Here's how the part is built. I have some questions about the finished solid (model axes, mm). A direction names the side the tool comes from. Round coordinates to 2 decimals unless told otherwise and drop trailing zeros. Loops run counter-clockwise (first coordinate to the right, second up) from the corner with the lowest first, then second, coordinate; pieces in that order, holes last. Notation, with made-up numbers: M 62.25,27.5 L 85.25,27.5 A17 cw 85.25,45.5 Z; hole C 65,21.25 d1. An arc over 180 degrees is marked long. Answer as a JSON object with one key per item and string values.
Autodesk Inventor part; units mm, degrees
ref_plane "YZ Plane" through (0, 0, 0) normal (1, 0, 0) x (0, 1, 0)
ref_plane "XZ Plane" through (0, 0, 0) normal (0, 1, 0) x (-1, 0, 0)
ref_plane "XY Plane" through (0, 0, 0) normal (0, 0, 1) x (1, 0, 0)
sketch "Sketch1" plane through (0, 0, 0) normal (0, 1, 0) x (-1, 0, 0)
  line L0 (-10, -20) -> (10, -20)
  line L1 (10, -20) -> (10, 20)
  line L2 (10, 20) -> (-10, 20)
  line L3 (-10, 20) -> (-10, -20)
  line L4 (-10, -20) -> (10, 20) construction
  line L5 (10, -20) -> (-10, 20) construction
  point P0 (0, 0)
  dimension "d0" = 20
  dimension "d1" = 40
extrude "Extrusion1" add sketch "Sketch1" along normal blind 60
sketch "Sketch2" plane through (0, 0, 0) normal (0, -1, 0) x (1, 0, 0)
  line L0 (10, -20) -> (-10, -20)
  line L1 (10, 20) -> (10, -20)
  line L2 (-10, 20) -> (10, 20)
  line L3 (-10, -20) -> (-10, 20)
  line L4 (10, 20) -> (10, -20)
  line L5 (10, 18.3) -> (-5.8, 18.3)
  line L6 (-5.8, 18.3) -> (-5.8, 16.1)
  line L7 (-5.8, 16.1) -> (10, 16.1)
  line L8 (10, 16.1) -> (10, 18.3)
  point P0 (0, 0)
  dimension "d4" = 1.7
  dimension "d5" = 4.2
  dimension "d6" = 2.2
extrude "Extrusion2" cut sketch "Sketch2" against normal through all contours L7 L6 L5 L1
mirror "Mirror1" about plane through (0, 0, 0) normal (0, 0, 1) of "Extrusion2"
sketch "Sketch3" plane through (0, 0, 0) normal (0, -1, 0) x (1, 0, 0)
  line L0 (-5.8, -16.1) -> (10, -16.1)
  line L1 (10, 16.1) -> (10, -16.1)
  line L2 (10, 16.1) -> (-5.8, 16.1)
  line L3 (-5.8, 16.1) -> (-5.8, 18.3)
  line L4 (-5.8, 18.3) -> (10, 18.3)
  line L5 (10, 20) -> (10, 18.3)
  line L6 (-10, 20) -> (10, 20)
  line L7 (-10, -20) -> (-10, 20)
  line L8 (10, -20) -> (-10, -20)
  line L9 (10, -18.3) -> (10, -20)
  line L10 (10, -18.3) -> (-5.8, -18.3)
  line L11 (-5.8, -18.3) -> (-5.8, -16.1)
  line L12 (10, 14.8) -> (-5.8, 14.8)
  line L13 (-5.8, 14.8) -> (-5.8, 12.28)
  line L14 (-5.8, 12.28) -> (10, 12.28)
  line L15 (10, 12.28) -> (10, 14.8)
  point P0 (0, 0)
  dimension "d9" = 1.3
  dimension "d10" = 2.52
extrude "Extrusion3" cut sketch "Sketch3" against normal through all contours L14 L13 L12 L1
pattern_linear "Rectangular Pattern1" count 8 spacing 3.82 along (0, 0, -1) of "Extrusion3"
sketch "Sketch4" plane through (-10, 0, 20) normal (0, 0, 1) x (1, 0, 0)
  line L0 (-20.7139, 77.7692) -> (45.2661, 77.7692)
  line L1 (45.2661, 77.7692) -> (45.2661, -19.6204)
  line L2 (45.2661, -19.6204) -> (-20.7139, -19.6204)
  line L3 (-20.7139, -19.6204) -> (-20.7139, 77.7692)
  point P0 (10, 0)
extrude "Extrusion4" cut sketch "Sketch4" against normal up to surface (15.36 mm away)
sketch "Sketch5" plane through (10, 0, 4.64) normal (1, 0, 0) x (0, 0, -1)
  line L0 (-2.9581, -8.043) -> (28.5295, -8.043)
  line L1 (28.5295, -8.043) -> (28.5295, 70.3336)
  line L2 (28.5295, 70.3336) -> (-2.9581, 70.3336)
  line L3 (-2.9581, 70.3336) -> (-2.9581, -8.043)
  point P0 (4.64, 0)
extrude "Extrusion5" cut sketch "Sketch5" against normal blind 4
properties part number "Jetson_Heatsink"
Item 1: We'd pull the mould along Z, two halves only. Please class faces 1 (the face through (-3.7, 60, -7.5)), 2 (the face through (0, 30, -0.48)), 3 (the face through (-2, 30, 4.64)), 4 (the face through (-2, 30, -20)): +Z half, -Z half, draft (parallel to the pull), parting line (faces both ways), or undercut.
Solution:
{"face 1": "draft", "face 2": "undercut", "face 3": "+Z half", "face 4": "-Z half"}
Item 2: I want a section at A-A on x = -2.25. List the corners of the cut face in (y, z) for me, plus the area to 3 significant figures.
Solution:
{"outline": "M 0,-20 L 60,-20 L 60,-18.3 L 0,-18.3 Z; M 0,-16.1 L 60,-16.1 L 60,-14.46 L 0,-14.46 Z; M 0,-11.94 L 60,-11.94 L 60,-10.64 L 0,-10.64 Z; M 0,-8.12 L 60,-8.12 L 60,-6.82 L 0,-6.82 Z; M 0,-4.3 L 60,-4.3 L 60,-3 L 0,-3 Z; M 0,-0.48 L 60,-0.48 L 60,0.82 L 0,0.82 Z; M 0,3.34 L 60,3.34 L 60,4.64 L 0,4.64 Z", "area": "590 mm2"}
Item 3: If I drill on L1, parallel to X at y = 52.5, z = -12.5, over which ranges is the centre line in solid material (lowest first)? Write a range as from..to.
Solution:
{"L1": "x = -10..-5.8"}
Item 4: For faces 5 (the face through (6, 30, -19)), 6 (the face through (-5.8, 30, -13)), which set-ups out of +Z, -Z, +X, -X, +Y, -Y let a thin tool reach every point of the face, with its end or its side?
Solution:
{"face 5": "+Z, -Z, +X, +Y, -Y", "face 6": "+X, +Y, -Y"}
Item 5: I want a section at C-C on z = 2.25. List the corners of the cut face in (x, y) for me, plus the area to 3 significant figures.
Solution:
{"outline": "M -10,0 L -5.8,0 L -5.8,60 L -10,60 Z", "area": "252 mm2"}
Item 6: I want a section at B-B on y = 34.5. List the corners of the cut face in (x, z) for me, plus the area to 3 significant figures.
Solution:
{"outline": "M -10,-20 L 6,-20 L 6,-18.3 L -5.8,-18.3 L -5.8,-16.1 L 6,-16.1 L 6,-14.46 L -5.8,-14.46 L -5.8,-11.94 L 6,-11.94 L 6,-10.64 L -5.8,-10.64 L -5.8,-8.12 L 6,-8.12 L 6,-6.82 L -5.8,-6.82 L -5.8,-4.3 L 6,-4.3 L 6,-3 L -5.8,-3 L -5.8,-0.48 L 6,-0.48 L 6,0.82 L -5.8,0.82 L -5.8,3.34 L 6,3.34 L 6,4.64 L -10,4.64 Z", "area": "220 mm2"}
Item 7: For P1, Ø0.7, axis at y = 29, z = -17, coming from the +X side, with a flat end and sliding along its axis, tell me the tip position at first contact or that it passes through.
Solution:
{"P1": "stops at x = -5.8"}
